Drawing for the job (mm, zero at the part's lowest x, y, z). A direction names the side the tool comes from. Round coordinates to 2 decimals unless told otherwise and drop trailing zeros. Write each loop counter-clockwise with the first axis right and the second up, starting at its lowest first coordinate (ties: lowest second). Pieces come first, ordered by that corner, then holes.
Item 1: Drop flat-ended pins along their axis: pin 1 Ø1 at (x, y) = (16, 14.5) entering from -Z; pin 2 Ø8 at (x, y) = (17.5, 12.5) entering from +Z; pin 3 Ø9 at (x, y) = (16.5, 27) entering from -Z; pin 4 Ø3.5 at (x, z) = (12, 28) entering from +Y. Give the stop position or say it passes through.
Item 2: Band-saw the part on A-A, the plane x = 15. Write the cut outline in (y, z), then the cut area to 4 significant figures.
Item 3: Wall check: probe 1 along Z at (x, y) = (23.25, 26.5); probe 2 along Y at (x, z) = (15, 8.85); probe 3 along Y at (x, z) = (21.75, 2.5). Give the ranges that are in metal, low to high.
Item 4: Band-saw the part on B-B, the plane y = 34. Write the cut outline in (x, z).
Item 5: Band-saw the part on C-C, the plane z = 6. Write the cut outline in (x, y), then the cut area to 3 significant figures.
Item 6: Mould opens along Y. For the marked faces 4, 5 and 6 say: +Y half, -Y half, draft (parallel to the pull), parting line (faces both ways), or undercut.
Item 7: 3-axis set-ups, long thin cutter, end or side, ignore diameter. For the marked faces 1, 2 and 3: which of +Z, -Z, +X, -X, +Y, -Y reach the whole face in a straight line?
Item 8: Band-saw the part on D-D, the plane x = 25.5. Write the cut outline in (y, z), then the cut area to 4 significant figures.
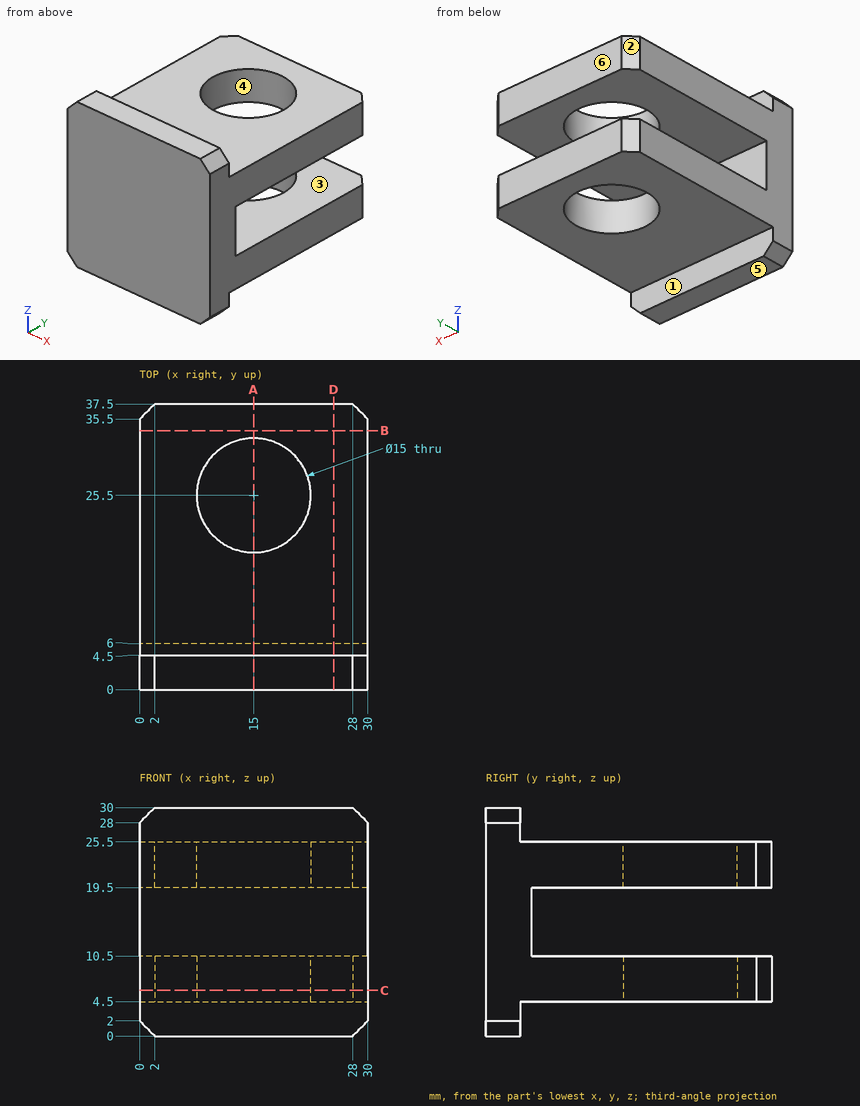
Results:
1. pin 1: stops at z = 4.5
1. pin 2: stops at z = 25.5
1. pin 3: passes through
1. pin 4: stops at y = 4.5
2. outline: (0, 0) - (4.5, 0) - (4.5, 4.5) - (18, 4.5) - (18, 10.5) - (6, 10.5) - (6, 19.5) - (18, 19.5) - (18, 25.5) - (4.5, 25.5) - (4.5, 30) - (0, 30) - close; (33, 4.5) - (37.5, 4.5) - (37.5, 10.5) - (33, 10.5) - close; (33, 19.5) - (37.5, 19.5) - (37.5, 25.5) - (33, 25.5) - close
2. area: 364.5 mm2
3. probe 1: z = 4.5 to 10.5, 19.5 to 25.5
3. probe 2: y = 0 to 18, 33 to 37.5
3. probe 3: y = 0 to 4.5
4. outline: (0, 4.5) - (30, 4.5) - (30, 10.5) - (0, 10.5) - close; (0, 19.5) - (30, 19.5) - (30, 25.5) - (0, 25.5) - close
5. outline: (0, 0) - (30, 0) - (30, 35.5) - (28, 37.5) - (2, 37.5) - (0, 35.5) - close; hole circle Ø15 at (15, 25.5)
5. area: 944 mm2
6. face 4: undercut
6. face 5: draft
6. face 6: +Y half
7. face 1: -Z, +X, -X, +Y
7. face 2: +Z, -Z, -X, +Y
7. face 3: +X, -X, +Y
8. outline: (0, 0) - (4.5, 0) - (4.5, 4.5) - (37.5, 4.5) - (37.5, 10.5) - (6, 10.5) - (6, 19.5) - (37.5, 19.5) - (37.5, 25.5) - (4.5, 25.5) - (4.5, 30) - (0, 30) - close
8. area: 544.5 mm2
